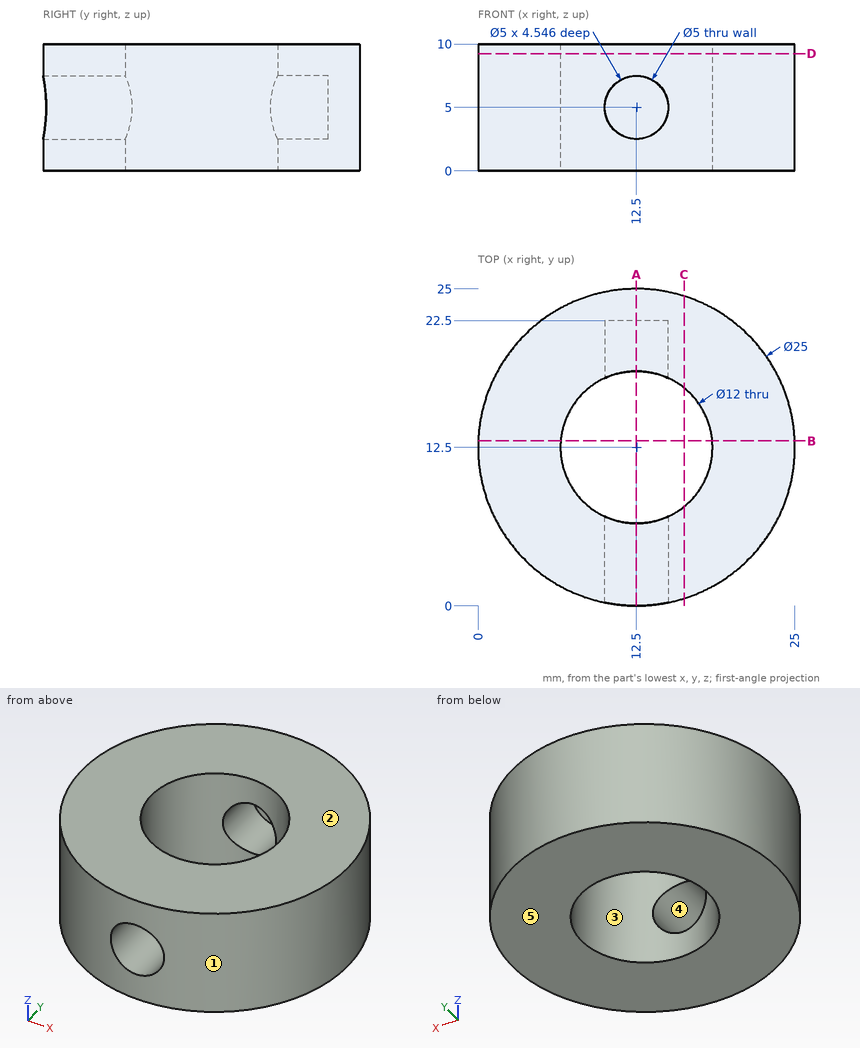
Can you work these out from the drawing? Everything is in mm from the part's minimum corner. A direction names the side the tool comes from. Give positions to 0.01 mm unless a question says otherwise; leave off trailing zeros. Order: outer loops, then holes, each group sorted by start corner. A loop starts at its lowest first (then second) coordinate and runs counter-clockwise, first axis right, second up. Notation, with made-up numbers: M -36,-36.75 L 10,-36.75 A11 ccw 10,-26.75 Z; hole C 44,64 d1. An arc over 180 degrees is marked long. Use a Markdown table: item, result. Add a question column.
Item 1: Will these pins go through, and if not, where does the flat tip stop? pin 1 (5 mm diameter, centred on x = 9, z = 4, fed in from -Y); pin 2 (6 mm diameter, centred on x = 21, z = 6, fed in from +Y) (1 decimal); pin 3 (6 mm diameter, centred on y = 16, z = 2, fed in from +X).
Item 2: For the marked faces 4 and 5, which set-ups out of +Z, -Z, +X, -X, +Y, -Y let a thin tool reach every point of the face, with its end or its side?
Item 3: We'd pull the mould along Y, two halves only. Please class the marked faces 1, 2 and 3: +Y half, -Y half, draft (parallel to the pull), parting line (faces both ways), or undercut.
Item 4: Suppose I cut it at B-B (y = 13). List the corners of the cut face in (x, z) for me.
Item 5: Suppose I cut it at D-D (z = 9.25). List the corners of the cut face in (x, y) for me.
Item 6: If I drill on L1, parallel to Z at x = 12.5, y = 1.5; L2, parallel to X at y = 11.25, z = 4.5; L3, parallel to X at y = 20, z = 4, over which ranges is the centre line in solid material (lowest first)? Write a range as [from, to].
Item 7: Suppose I cut it at A-A (x = 12.5). List the corners of the cut face in (y, z) for me.
Item 8: Suppose I cut it at C-C (x = 16.25). List the corners of the cut face in (y, z) for me.
Answer sheet:
| question | item | result |
|---|---|---|
| 1 | pin 1 | stops at y = 0.07 |
| 1 | pin 2 | stops at y = 23.7 |
| 1 | pin 3 | stops at x = 24.99 |
| 2 | face 4 | -Y |
| 2 | face 5 | -Z, +X, -X, +Y, -Y |
| 3 | face 1 | parting line |
| 3 | face 2 | draft |
| 3 | face 3 | undercut |
| 4 | outline | M 0.01,0 L 6.52,0 L 6.52,10 L 0.01,10 Z; M 18.48,0 L 24.99,0 L 24.99,10 L 18.48,10 Z |
| 5 | outline | C 12.5,12.5 d25; hole C 12.5,12.5 d12 |
| 6 | L1 | z = [0, 2.5], [7.5, 10] |
| 6 | L2 | x = [0.06, 6.63], [18.37, 24.94] |
| 6 | L3 | x = [2.5, 10.21], [14.79, 22.5] |
| 7 | outline | M 0,0 L 6.5,0 L 6.5,2.5 L 0,2.5 Z; M 0,7.5 L 6.5,7.5 L 6.5,10 L 0,10 Z; M 18.5,0 L 25,0 L 25,10 L 18.5,10 L 18.5,7.5 L 22.5,7.5 L 22.5,2.5 L 18.5,2.5 Z |
| 8 | outline | M 0.58,0 L 7.82,0 L 7.82,10 L 0.58,10 Z; M 17.18,0 L 24.42,0 L 24.42,10 L 17.18,10 Z |
